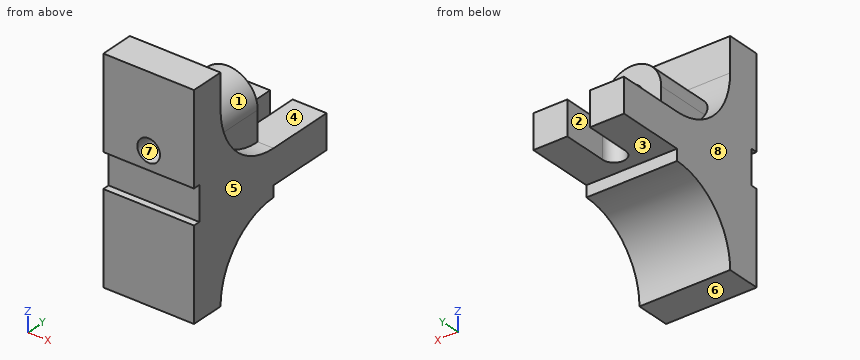
from build123d import *

# Parameters (mm, degrees)
BOSS_EXTRUDE4_DEPTH      = 20
BOSS_EXTRUDE5_REACH      = 70.42
BOSS_EXTRUDE5_END_RADIUS = 30
SKETCH7_R                = 5
CUT_EXTRUDE1_DEPTH       = 69.419660946
SKETCH8_W                = 15
SKETCH8_H                = 30
BOSS_EXTRUDE6_DEPTH      = 40
CUT_EXTRUDE2_REACH       = 94.331


with BuildPart() as part:
    # Sketch1 → Boss-Extrude4 (new, symmetric)
    with BuildSketch(Plane(origin=(0, 0, 0), x_dir=(0, 0, -1), z_dir=(1, 0, 0))):
        with BuildLine():
            Line((-47.5, 0), (-7.5, 0))
            Line((-7.5, 0), (-7.5, 3))
            Line((-7.5, 3), (7.5, 3))
            Line((7.5, 3), (7.5, 0))
            Line((7.5, 0), (47.5, 0))
            Line((47.5, 0), (47.5, 15))
            ThreePointArc((47.5, 15), (26.286796564, 23.786796564), (17.5, 45))
            Line((17.5, 45), (12.5, 45))
            Line((12.5, 45), (-2.5, 45))
            ThreePointArc((-2.5, 45), (-11.286796564, 23.786796564), (-32.5, 15))
            Line((-32.5, 15), (-47.5, 15))
            Line((-47.5, 15), (-47.5, 0))
        make_face()
    extrude(amount=BOSS_EXTRUDE4_DEPTH, both=True)

    # Boss-Extrude5: up to this cylinder (the profile starts inside it)
    boss_extrude5_end = Plane(origin=(0, 45, 32.5), z_dir=(-1, 0, 0)) * Cylinder(BOSS_EXTRUDE5_END_RADIUS, 201.84, mode=Mode.PRIVATE)
    # Sketch6 → Boss-Extrude5 (add, up to the surface)
    with BuildSketch(Plane(origin=(0, 45, 0), x_dir=(1, 0, 0), z_dir=(0, 1, 0)), mode=Mode.PRIVATE) as boss_extrude5_sk1:
        with BuildLine():
            Line((-13, -15.5), (-13, -2.5))
            Line((-13, -2.5), (13, -2.5))
            Line((13, -2.5), (13, -15.5))
            ThreePointArc((13, -15.5), (0, -28.5), (-13, -15.5))
        make_face()
    boss_extrude5_tool1 = extrude(boss_extrude5_sk1.sketch, amount=-BOSS_EXTRUDE5_REACH, mode=Mode.PRIVATE) & boss_extrude5_end
    add(boss_extrude5_tool1.solids().sort_by_distance((0, 45, 14.286452))[0])

    # Sketch7 → Cut-Extrude1 (cut, through all)
    with BuildSketch(Plane(origin=(0, 45, 0), x_dir=(1, 0, 0), z_dir=(0, 1, 0))):
        with Locations(Location((0, -15.5, 0), (0, 0, 270))):
            Circle(SKETCH7_R)
    extrude(amount=-CUT_EXTRUDE1_DEPTH, mode=Mode.SUBTRACT)

    # Sketch8 → Boss-Extrude6 (add)
    with BuildSketch(Plane(origin=(20, 0, 0), x_dir=(0, 0, -1), z_dir=(1, 0, 0))):
        with Locations((5, 60)):
            Rectangle(SKETCH8_W, SKETCH8_H)
    extrude(amount=-BOSS_EXTRUDE6_DEPTH)

    # Sketch9 → Cut-Extrude2 (cut, up to next)
    with BuildSketch(Plane.XY.offset(2.5), mode=Mode.PRIVATE) as cut_extrude2_sk1:
        with BuildLine():
            Line((-5, 75), (5, 75))
            Line((5, 75), (5, 55))
            ThreePointArc((5, 55), (0, 50), (-5, 55))
            Line((-5, 55), (-5, 75))
        make_face()
    cut_extrude2_tool1 = extrude(cut_extrude2_sk1.sketch, amount=-CUT_EXTRUDE2_REACH, mode=Mode.PRIVATE) & part.part
    add(cut_extrude2_tool1.solids().sort_by_distance((0, 63.010479, 2.5))[0], mode=Mode.SUBTRACT)


solid = part.part
Work out the finished part from the listing and answer in its coordinate system (mm). Face numbers are marked on the shaded views. A direction names the side the tool comes from. Give positions to 0.01 mm unless a question says otherwise; leave off trailing zeros. Write each loop counter-clockwise with the first axis right and the second up, starting at its lowest first coordinate (ties: lowest second). Pieces come first, ordered by that corner, then holes.
Q1. The part is cut by section B-B on y = 61.5. Give the vertices of the cut face in (x, z), and give its area (3 significant figures).
Answer:
outline: (-20, -12.5) - (-5, -12.5) - (-5, 2.5) - (-20, 2.5) - close; (5, -12.5) - (20, -12.5) - (20, 2.5) - (5, 2.5) - close
area: 450 mm2
Q2. The part is cut by section D-D on y = 43. Give the vertices of the cut face in (x, z).
Answer:
outline: (-20, -17.57) - (20, -17.57) - (20, 2.57) - (13, 2.57) - (13, 15.5) arc R13 ccw to (-13, 15.5) - (-13, 2.57) - (-20, 2.57) - close; hole circle Ø10 at (0, 15.5)
Q3. Given pin 1 (1 mm diameter, centred on x = 6.5, z = 24.5, fed in from -Y); pin 2 (4 mm diameter, centred on y = 36, z = 10, fed in from +X); pin 3 (24 mm diameter, centred on x = -10, y = 66, fed in from +Z); pin 4 (12 mm diameter, centred on x = 7, z = 11, fed in from +Y), each flat-ended and moving along its own axis, determine where each tip first touches the part or whether it passes through.
Answer:
pin 1: stops at y = 0
pin 2: stops at x = 13
pin 3: stops at z = 2.5
pin 4: stops at y = 45
Q4. The part is cut by section A-A on x = 0. Give the vertices of the cut face in (y, z).
Answer:
outline: (0, -47.5) - (15, -47.5) arc R30 cw to (45, -17.5) - (45, -12.5) - (50, -12.5) - (50, 2.5) - (45, 2.5) - (45, 10.5) - (0, 10.5) - (0, 7.5) - (3, 7.5) - (3, -7.5) - (0, -7.5) - close; (0, 20.5) - (45, 20.5) - (45, 28.5) - (15.27, 28.5) arc R30 cw to (15, 32.5) - (15, 47.5) - (0, 47.5) - close
Q5. Straight lines are drawn through the part: L1, parallel to X at y = 29, z = 15; L2, parallel to Y at x = -4.5, z = 4.5; L3, parallel to Y at x = 17, z = 35. For each, find the intervals that lie inside material, in ascending order.
Answer:
L1: x = -13 to -4.97, 4.97 to 13
L2: y = 3 to 45
L3: y = 0 to 15
Q6. A tool of negligible diameter and unlimited length cuts with its end or side. For the marked faces 1, 2, 3 and 4, from which of +Z, -Z, +X, -X, +Y, -Y can it reach the whole face along a straight path? Write none if from no direction.
Answer:
face 1: +Z, +Y
face 2: +Z, -Z, +Y
face 3: -Z, +X, -X, +Y
face 4: +Z, +X, -X, +Y
Q7. For a pull along X with two mould halves and no side action, classify the marked faces 5, 6, 7 and 8 as released by +X, released by -X, zero draft, split by the parting line, or undercut.
Answer:
face 5: released by +X
face 6: zero draft
face 7: undercut
face 8: released by -X
Q8. The part is cut by section C-C on z = -0.5. Give the vertices of the cut face in (x, y).
Answer:
outline: (-20, 3) - (20, 3) - (20, 75) - (5, 75) - (5, 55) arc R5 cw to (-5, 55) - (-5, 75) - (-20, 75) - close
